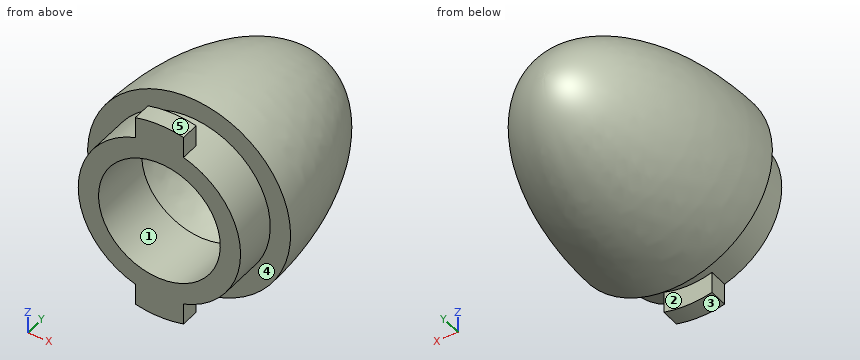
```python
from build123d import *

# Parameters (mm, degrees)
BOSS_EXTRUDE1_START = 2.54
BOSS_EXTRUDE1_DEPTH = 1.905


with BuildPart() as part:
    # Sketch1 → Revolve1 (revolve)
    with BuildSketch(Plane(origin=(0, 0, 0), x_dir=(0, 0, -1), z_dir=(1, 0, 0)), mode=Mode.PRIVATE) as revolve1_sk:
        with BuildLine():
            Line((-8.128, 0), (-8.128, 4.445))
            Line((-8.128, 4.445), (-10.16, 4.445))
            add(Edge.make_bspline(
                [(0, 23.495), (-10.16, 23.495), (-10.16, 4.445)],
                knots=[3.141592654, 3.141592654, 3.141592654, 4.71238898, 4.71238898, 4.71238898], degree=2, weights=[1, 0.707106781, 1]))
            Line((0, 23.495), (0, 21.463))
            add(Edge.make_bspline(
                [(0, 21.463), (-0.398270959, 21.463), (-1.153389942, 21.335826731), (-2.429445225, 20.684705062), (-3.759980482, 19.474733116), (-5.045566653, 17.699172098), (-6.18547282, 15.416687429), (-7.108495403, 12.712906185), (-7.763293706, 9.707759052), (-8.001641772, 7.545168518), (-8.066508555, 6.477)],
                knots=[3.141592654, 3.141592654, 3.141592654, 3.141592654, 3.323770314, 3.505947975, 3.688125635, 3.870303296, 4.052480956, 4.234658617, 4.416836277, 4.599013938, 4.599013938, 4.599013938, 4.599013938], degree=3))
            Line((-8.066508555, 6.477), (-6.096, 6.477))
            Line((-6.096, 6.477), (-6.096, 0))
            Line((-6.096, 0), (-8.128, 0))
        make_face()
    revolve(revolve1_sk.sketch.rotate(Axis((0, 0, 0), (0, 1, 0)), 180), axis=Axis((0, 0, 0), (0, 1, 0)))

    # Sketch2 → Boss-Extrude1 (add)
    with BuildSketch(Plane.XZ.offset(-4.445).offset(BOSS_EXTRUDE1_START)):
        with BuildLine():
            Line((-2.413, 9.869297391), (-2.413, 7.761560088))
            ThreePointArc((-2.413, 7.761560088), (0, 8.128), (2.413, 7.761560088))
            Line((2.413, 7.761560088), (2.413, 9.869297391))
            ThreePointArc((2.413, 9.869297391), (0, 10.16), (-2.413, 9.869297391))
        make_face()
        with BuildLine():
            Line((2.413, -9.869297391), (2.413, -7.761560088))
            ThreePointArc((2.413, -7.761560088), (0, -8.128), (-2.413, -7.761560088))
            Line((-2.413, -7.761560088), (-2.413, -9.869297391))
            ThreePointArc((-2.413, -9.869297391), (0, -10.16), (2.413, -9.869297391))
        make_face()
    extrude(amount=BOSS_EXTRUDE1_DEPTH)


solid = part.part
```
For this review, take the finished solid that the model builds, in its own axes (mm). Face numbers are marked on the shaded views. A direction names the side the tool comes from. Coordinates: 2 decimals unless noted, no trailing zeros. Return JSON: item names as keys, results as strings. Group by question number.
(1) For pin 1 Ø2 at (y, z) = (1, -9) entering from -X; pin 2 Ø12 at (y, z) = (6, -1.5) entering from -X; pin 3 Ø1 at (y, z) = (1, -9) entering from +X; pin 4 Ø5 at (y, z) = (9, 8) entering from -X, all flat-tipped, find the tip position at first contact; note any pin that passes through.
(2) Mouldability with a two-part tool opening along Z and no side actions: class the marked faces 1, 2 and 3 as pulls with the +Z half, pulls with the -Z half, needs draft (parallel to the pull), parting line crosses it, or undercut.
(3) To check wall thickness, follow L1, parallel to X at y = 1.5, z = 0; L2, parallel to X at y = 5, z = 0; L3, parallel to Z at x = -4.75, y = 14. State the ranges of each line that lie inside material, in increasing order.
(4) Tool access review of the marked faces 4 and 5: name each direction out of +Z, -Z, +X, -X, +Y, -Y from which nothing blocks a thin tool from reaching the whole face with its end or side.
Results below:
{
 "1": {"pin 1": "stops at x = -2.41", "pin 2": "stops at x = -10.16", "pin 3": "stops at x = 2.41", "pin 4": "stops at x = -8.23"},
 "2": {"face 1": "undercut", "face 2": "needs draft", "face 3": "pulls with the -Z half"},
 "3": {"L1": "x = -8.13 to -6.1, 6.1 to 8.13", "L2": "x = -10.16 to -6.1, 6.1 to 10.16", "L3": "z = -7.4 to -4.66, 4.66 to 7.4"},
 "4": {"face 4": "none", "face 5": "+Z, +Y, -Y"}
}
